```python
from build123d import *

# Parameters (mm, degrees)
SKETCH3_R          = 0.685
CUT_EXTRUDE1_DEPTH = 1.17
SKETCH4_R          = 0.875
CUT_EXTRUDE2_DEPTH = 0.6
CIRPATTERN1_COUNT  = 3
SCALE1_SCALE       = 10
CUT_EXTRUDE3_DEPTH = 4
SKETCH8_R          = 1.45
CUT_EXTRUDE4_DEPTH = 10


with BuildPart() as part:
    # Sketch1 → Revolve1 (revolve)
    with BuildSketch(Plane.XY):
        with BuildLine():
            Line((0, 0), (-6, 0))
            add(Edge.make_bspline(
                [(-6, 0), (-6, 1.777820911), (-4.715943748, 2), (0, 2)],
                knots=[0, 0, 0, 0, 1, 1, 1, 1], degree=3))
            Line((0, 2), (0, 0))
        make_face()
    revolve(axis=Axis((0, 0, 0), (-1, 0, 0)))

    # Sketch3 → Cut-Extrude1 (cut)
    with BuildSketch(Plane.XY.offset(2)):
        with Locations((-3.5, 0)):
            Circle(SKETCH3_R)
    cut_extrude1 = extrude(amount=-CUT_EXTRUDE1_DEPTH, mode=Mode.SUBTRACT)

    # Sketch4 → Cut-Extrude2 (cut)
    with BuildSketch(Plane.XY.offset(2)):
        with Locations((-3.5, 0)):
            Circle(SKETCH4_R)
    cut_extrude2 = extrude(amount=-CUT_EXTRUDE2_DEPTH, mode=Mode.SUBTRACT)

    # CirPattern1: Cut-Extrude1, Cut-Extrude2 ×3 about axis
    cirpattern1_axis = Axis((0, 0, 0), (1, 0, 0))
    add([cut_extrude1.rotate(cirpattern1_axis, i * 360 / CIRPATTERN1_COUNT) for i in range(1, CIRPATTERN1_COUNT)], mode=Mode.SUBTRACT)
    add([cut_extrude2.rotate(cirpattern1_axis, i * 360 / CIRPATTERN1_COUNT) for i in range(1, CIRPATTERN1_COUNT)], mode=Mode.SUBTRACT)


with BuildPart() as part_1:
    # Scale1: scaled about (-2.513849937, -2.1e-08, 6.5e-08)
    add(part.part.scale(SCALE1_SCALE).moved(Location((22.624649433, 1.89e-07, -5.85e-07))))

    # Sketch7 → Cut-Extrude3 (cut)
    with BuildSketch(Plane(origin=(22.625249359, 0, 0), x_dir=(0, 0, -1), z_dir=(1, 0, 0))):
        Polygon((0, 8.717989065), (-7.55, 4.358994532), (-7.55, -4.358994532), (0, -8.717989065), (7.55, -4.358994532), (7.55, 4.358994532), align=None)
    extrude(amount=-CUT_EXTRUDE3_DEPTH, mode=Mode.SUBTRACT)

    # Sketch8 → Cut-Extrude4 (cut)
    with BuildSketch(Plane(origin=(22.625249359, 0, 0), x_dir=(0, 0, -1), z_dir=(1, 0, 0))):
        with Locations(Location((-7, 12.5, 0), (0, 0, 90))):
            Circle(SKETCH8_R)
        with Locations(Location((14.325317547, -0.187822174, 0), (0, 0, 90))):
            Circle(SKETCH8_R)
        with Locations(Location((-7.325317547, -12.312177826, 0), (0, 0, 90))):
            Circle(SKETCH8_R)
    extrude(amount=-CUT_EXTRUDE4_DEPTH, mode=Mode.SUBTRACT)


solid = part_1.part
```
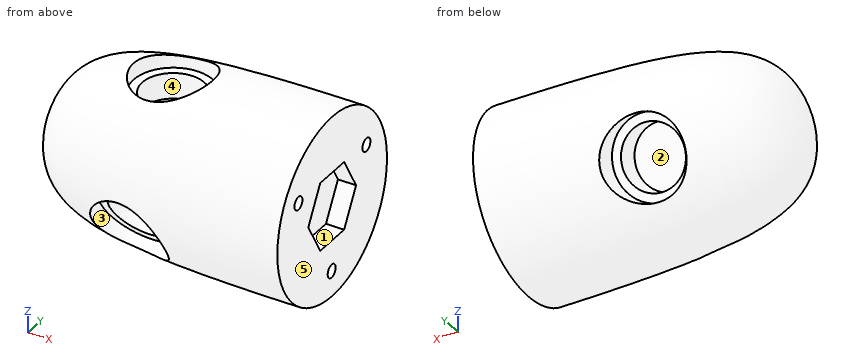
Geometry check sheet. Reference: the model listing, model coordinates, mm. Face numbers are marked on the shaded views. A direction names the side the tool comes from. Give positions to 0.01 mm unless a question says otherwise; leave off trailing zeros. Write item = value, one per line. Start each with the question number.
1. Go/stop test with flat-tipped pins: P1, Ø3, axis at x = 5, z = -5, coming from the -Y side; P2, Ø12, axis at x = -20, z = 9.5, coming from the +Y side; P3, Ø2, axis at x = -26, y = -9, coming from the +Z side. Record where each tip stops, or that it passes through.
2. Tool access check on the marked faces 1 and 2. Record the directions out of +Z, -Z, +X, -X, +Y, -Y that give a thin tool (end or side, any length) a straight path to the whole face; none if there is none.
3. Thickness scan on probe 1 along Y at (x, z) = (16, 7.5); probe 2 along Y at (x, z) = (13.5, 12.5); probe 3 along Z at (x, y) = (-15, -9). Record the ranges inside material, lowest first.
4. Draft check along Y on the marked faces 3, 4 and 5. Enter one of: +Y half, -Y half, draft (parallel to the pull), parting line (faces both ways), or undercut.
Values follow:
q1.P1 = -19.53
q1.P2 = 17.86
q1.P3 = 14.39
q2.face_1 = +X
q2.face_2 = none
q3.probe_1 = -18.52 to -13.75, -10.87 to 11.14, 13.86 to 18.52
q3.probe_2 = -15.57 to 15.57
q3.probe_3 = -16.32 to -14.83, -1.01 to 16.32
q4.face_3 = undercut
q4.face_4 = undercut
q4.face_5 = draft
